Source: CAD feature listing. Evaluate the final solid. Frame: model axes, mm. A direction names the side the tool comes from. Give positions to 0.01 mm unless a question says otherwise; leave off trailing zeros. Loops run counter-clockwise (first coordinate to the right, second up) from the corner with the lowest first, then second, coordinate; pieces in that order, holes last. Notation, with made-up numbers: M 17.5,18.25 L 48.5,18.25 A20 cw 48.5,49.25 Z; hole C -31.75,-19.75 d6. An arc over 180 degrees is marked long. Answer in a Markdown table with one row per item.
```python
from build123d import *

# Parameters (mm, degrees)
SZKIC1_W                    = 66.5
SZKIC1_H                    = 42.8
DODANIE_WYCI_GNI_CIE1_DEPTH = 5.4
SZKIC2_W                    = 53.5
SZKIC2_H                    = 29.8
WYTNIJ_WYCI_GNI_CIE1_DEPTH  = 120.279744778
SZKIC3_R                    = 1.6
WYTNIJ_WYCI_GNI_CIE2_DEPTH  = 10
SZKIC5_W                    = 5.5
SZKIC5_H                    = 1
DODANIE_WYCI_GNI_CIE2_DEPTH = 29.8
SZKIC6_W                    = 4
SZKIC6_H                    = 1
DODANIE_WYCI_GNI_CIE3_DEPTH = 4
SZKIC7_W                    = 4
SZKIC7_H                    = 1
DODANIE_WYCI_GNI_CIE4_DEPTH = 4
SZKIC8_W                    = 7.080014019
SZKIC8_H                    = 1
DODANIE_WYCI_GNI_CIE5_DEPTH = 3
SZKIC9_W                    = 7.08
SZKIC9_H                    = 1
DODANIE_WYCI_GNI_CIE6_DEPTH = 3


with BuildPart() as part:
    # Szkic1 → Dodanie-wyciągnięcie1 (new body)
    with BuildSketch(Plane.XY):
        with Locations((-69.098753826, 39.618276807)):
            Rectangle(SZKIC1_W, SZKIC1_H)
    extrude(amount=DODANIE_WYCI_GNI_CIE1_DEPTH)

    # Szkic2 → Wytnij-wyciągnięcie1 (cut, through all)
    with BuildSketch(Plane.XY.offset(5.4)):
        with Locations((-69.098753826, 39.618276807)):
            Rectangle(SZKIC2_W, SZKIC2_H)
    extrude(amount=-WYTNIJ_WYCI_GNI_CIE1_DEPTH, mode=Mode.SUBTRACT)

    # Szkic3 → Wytnij-wyciągnięcie2 (cut)
    with BuildSketch(Plane.XY.offset(5.4)):
        with Locations((-99.098753826, 57.768276807)):
            Circle(SZKIC3_R)
        with Locations((-39.098753826, 57.768276807)):
            Circle(SZKIC3_R)
        with Locations((-39.098753826, 21.468276807)):
            Circle(SZKIC3_R)
        with Locations((-99.098753826, 21.468276807)):
            Circle(SZKIC3_R)
    extrude(amount=-WYTNIJ_WYCI_GNI_CIE2_DEPTH, mode=Mode.SUBTRACT)

    # Szkic5 → Dodanie-wyciągnięcie2 (add)
    with BuildSketch(Plane.XZ.offset(-54.518276807)):
        with Locations((-77.598753826, 4.9)):
            Rectangle(SZKIC5_W, SZKIC5_H)
    extrude(amount=DODANIE_WYCI_GNI_CIE2_DEPTH)

    # Szkic6 → Dodanie-wyciągnięcie3 (add)
    with BuildSketch(Plane.XZ.offset(-54.518276807)):
        with Locations((-44.348753826, 4.9)):
            Rectangle(SZKIC6_W, SZKIC6_H)
    extrude(amount=DODANIE_WYCI_GNI_CIE3_DEPTH)

    # Szkic7 → Dodanie-wyciągnięcie4 (add)
    with BuildSketch(Plane(origin=(0, 24.718276807, 0), x_dir=(1, 0, 0), z_dir=(0, 1, 0))):
        with Locations((-44.348753826, -4.9)):
            Rectangle(SZKIC7_W, SZKIC7_H)
    extrude(amount=DODANIE_WYCI_GNI_CIE4_DEPTH)

    # Szkic8 → Dodanie-wyciągnięcie5 (add)
    with BuildSketch(Plane.XZ.offset(-54.518276807)):
        with Locations((-92.308746817, 4.9)):
            Rectangle(SZKIC8_W, SZKIC8_H)
    extrude(amount=DODANIE_WYCI_GNI_CIE5_DEPTH)

    # Szkic9 → Dodanie-wyciągnięcie6 (add)
    with BuildSketch(Plane(origin=(0, 24.718276807, 0), x_dir=(1, 0, 0), z_dir=(0, 1, 0))):
        with Locations((-92.308753826, -4.9)):
            Rectangle(SZKIC9_W, SZKIC9_H)
    extrude(amount=DODANIE_WYCI_GNI_CIE6_DEPTH)


solid = part.part
```
1) Material intervals for L1, parallel to X at y = 39.5, z = 5; L2, parallel to X at y = 49, z = 4.1; L3, parallel to Y at x = -83.5, z = 5.2, sorted ascending.
Reply:
| item | result |
|---|---|
| L1 | x = -102.35 to -95.85, -80.35 to -74.85, -42.35 to -35.85 |
| L2 | x = -102.35 to -95.85, -42.35 to -35.85 |
| L3 | y = 18.22 to 24.72, 54.52 to 61.02 |
2) Pin query (flat end, axial travel): pin 1 Ø2 at (x, y) = (-44.5, 27) entering from -Z; pin 2 Ø2.5 at (x, y) = (-39.1, 57.77) entering from +Z. Return the tip coordinate at first contact, or that it passes through.
Reply:
| item | result |
|---|---|
| pin 1 | stops at z = 4.4 |
| pin 2 | passes through |
3) Set-up query: faces 1 (the flat face through (-70, 18.218, 3)), 2 (the flat face through (-92, 53, 4.4)). Return all of +Z, -Z, +X, -X, +Y, -Y with unobstructed straight access to the full face (end or side cutting, diameter ignored); none if empty.
Reply:
| item | result |
|---|---|
| face 1 | +Z, -Z, +X, -X, -Y |
| face 2 | -Z |
4) Pull-direction query (Y, two-part tool) for faces 3 (the flat face through (-42.349, 39, 3)), 4 (the flat face through (-70, 61.018, 3)), 5 (the flat face through (-77, 39, 5.4)); classes: released by +Y, released by -Y, zero draft, split by the parting line, or undercut.
Reply:
| item | result |
|---|---|
| face 3 | undercut |
| face 4 | released by +Y |
| face 5 | zero draft |
5) Section A-A, the plane y = 53.5. Return loops of the section in (x, z).
Reply:
| item | result |
|---|---|
| outline | M -102.35,0 L -95.85,0 L -95.85,4.4 L -88.77,4.4 L -88.77,5.4 L -102.35,5.4 Z; M -80.35,4.4 L -74.85,4.4 L -74.85,5.4 L -80.35,5.4 Z; M -46.35,4.4 L -42.35,4.4 L -42.35,0 L -35.85,0 L -35.85,5.4 L -46.35,5.4 Z |
6) Section B-B, the plane x = -83.5. Return loops of the section in (y, z).
Reply:
| item | result |
|---|---|
| outline | M 18.22,0 L 24.72,0 L 24.72,5.4 L 18.22,5.4 Z; M 54.52,0 L 61.02,0 L 61.02,5.4 L 54.52,5.4 Z |
7) Section D-D, the plane y = 46.5. Return loops of the section in (x, z).
Reply:
| item | result |
|---|---|
| outline | M -102.35,0 L -95.85,0 L -95.85,5.4 L -102.35,5.4 Z; M -80.35,4.4 L -74.85,4.4 L -74.85,5.4 L -80.35,5.4 Z; M -42.35,0 L -35.85,0 L -35.85,5.4 L -42.35,5.4 Z |
8) Section C-C, the plane z = 1.5. Return loops of the section in (x, y), then the cut area to 3 significant figures.
Reply:
| item | result |
|---|---|
| outline | M -102.35,18.22 L -35.85,18.22 L -35.85,61.02 L -102.35,61.02 Z; hole C -99.1,21.47 d3.2; hole C -99.1,57.77 d3.2; hole M -95.85,24.72 L -42.35,24.72 L -42.35,54.52 L -95.85,54.52 Z; hole C -39.1,21.47 d3.2; hole C -39.1,57.77 d3.2 |
| area | 1,220 mm² |
